Work out the finished part from the listing and answer in its coordinate system (mm). Face numbers are marked on the shaded views. A direction names the side the tool comes from. Give positions to 0.01 mm unless a question says otherwise; leave off trailing zeros. Loops run counter-clockwise (first coordinate to the right, second up) from the corner with the lowest first, then second, coordinate; pieces in that order, holes last. Notation, with made-up numbers: (-20.5, 16) - (16.5, 16) arc R21 cw to (16.5, 21) - close; hole circle Ø5 at (15.5, 85.5). An arc over 180 degrees is marked (long way). One line per question, with ' | ' between items. Start each with the question number.
1. Find the intervals of material crossed by line 1 (Y direction, x = 3.75, z = 0.65); line 2 (Y direction, x = 7.75, z = 1.4); line 3 (Y direction, x = 7.25, z = 2.8), in increasing order.
2. For a pull along Y with two mould halves and no side action, classify the marked faces 4, 5 and 6 as released by +Y, released by -Y, zero draft, split by the parting line, or undercut.
3. Which of the six approach directions +Z, -Z, +X, -X, +Y, -Y give full straight-line access (tool end or side, diameter ignored) to the marked faces 1, 2 and 3?
4. Section C-C (y = 9) is taken. Determine the outline of the cut face in (x, z).
5. Section A-A (x = 4) is taken. Determine the outline of the cut face in (y, z).
6. Section D-D (x = 0.25) is taken. Determine the outline of the cut face in (y, z).
7. Each of these flat-tipped pins is pushed along its axis until it touches: pin 1 (2 mm diameter, centred on x = -3, y = -3.5, fed in from +Z); pin 2 (1.5 mm diameter, centred on x = -6.5, z = 2, fed in from +Y); pin 3 (1.6 mm diameter, centred on y = -3.5, z = 1.5, fed in from +X). Where does it stop, or does it pass through?
Autodesk Inventor part; units mm, degrees
ref_plane "YZ Plane" through (0, 0, 0) normal (1, 0, 0) x (0, 1, 0)
ref_plane "XZ Plane" through (0, 0, 0) normal (0, 1, 0) x (-1, 0, 0)
ref_plane "XY Plane" through (0, 0, 0) normal (0, 0, 1) x (1, 0, 0)
sketch "Sketch1" plane through (0, 0, 0) normal (0, 0, 1) x (1, 0, 0)
  line L0 (-8.4, 0) -> (8.4, 0) construction
  line L1 (0, -20.65) -> (0, 20.65) construction
  line L2 (6, -14.75) -> (-6, -14.75)
  line L3 (-6, -14.75) -> (-6, 14.75)
  line L4 (-6, 14.75) -> (6, 14.75)
  line L5 (6, 14.75) -> (6, -14.75)
  line L6 (6, -14.75) -> (-6, 14.75) construction
  line L7 (-6, -14.75) -> (6, 14.75) construction
  point P0 (0, 0)
  dimension "d0" = 12
  dimension "d1" = 29.5
extrude "Extrusion1" add sketch "Sketch1" along normal blind 2
sketch "Sketch3" plane through (-6, 14.75, 2) normal (0, 1, 0) x (1, 0, 0)
  line L0 (0, 2) -> (12, 2) construction
  line L1 (0, 2) -> (0, 0) construction
  line L2 (12, 0) -> (0, 0) construction
  circle A0 centre (0, 0.5) radius 1.5
  line L3 (12, 2) -> (12, 0)
  point P0 (6, 2)
  dimension "d7" = 3
extrude "Extrusion3" add sketch "Sketch3" against normal up to surface (29.5 mm away)
sketch "Sketch5" plane through (6, 14.75, 2) normal (0, 1, 0) x (1, 0, 0)
  arc A0 (-12, 2) -> (-10.5858, 0) centre (-12, 0.5) ccw construction
  line L0 (0, 0) -> (-10.5858, 0) construction
  line L1 (0, 2) -> (0, 0) construction
  line L2 (-12, 2) -> (0, 2) construction
  circle A1 centre (-12, 0.5) radius 1.5
  point P0 (-6, 2)
extrude "Extrusion5" add sketch "Sketch5" along normal blind 1
mirror "Mirror3" about plane through (0, 0, 0) normal (0, 1, 0) of "Extrusion5"
sketch "Sketch6" plane through (0, 0, 2) normal (0, 0, 1) x (1, 0, 0)
  line L0 (-4.5858, 14.75) -> (-4.5858, -14.75) construction
  line L1 (-4.5858, -14.75) -> (6, -14.75) construction
  line L2 (6, -14.75) -> (6, 14.75) construction
  line L3 (6, 14.75) -> (-4.5858, 14.75) construction
  line L4 (-9.1, 0) -> (12.6, 0) construction
  line L5 (-6, 14.75) -> (6, 14.75)
  line L6 (1, 14.75) -> (1, 16.75)
  line L7 (1, 16.75) -> (10.5, 16.75)
  line L8 (2.75, 15.5) -> (2.75, 14.75)
  line L9 (1, 14.75) -> (2.75, 14.75)
  line L10 (2.75, 15.5) -> (6.75, 15.5)
  line L11 (6.75, 15.5) -> (6.75, 14.75)
  line L12 (6.75, 14.75) -> (10.5, 14.75)
  line L13 (10.5, 16.75) -> (10.5, 14.75)
  line L14 (6, 14.75) -> (-4.5858, 14.75)
  line L15 (1, -14.75) -> (1, -16.75)
  line L16 (1, -16.75) -> (10.5, -16.75)
  line L17 (2.75, -15.5) -> (2.75, -14.75)
  line L18 (1, -14.75) -> (2.75, -14.75)
  line L19 (2.75, -15.5) -> (6.75, -15.5)
  line L20 (6.75, -15.5) -> (6.75, -14.75)
  line L21 (6.75, -14.75) -> (10.5, -14.75)
  line L22 (10.5, -16.75) -> (10.5, -14.75)
  line L23 (0, 14.75) -> (0, 17.3845) construction
  point P0 (0, 0)
  dimension "d14" = 2
  dimension "d15" = 0.75
  dimension "d16" = 0.75
  dimension "d17" = 1.75
  dimension "d18" = 4.5
  dimension "d40" = 1
extrude "Extrusion6" add sketch "Sketch6" against normal up to surface (2 mm away)
sketch "Skizze9" plane through (0, 0, 2) normal (0, 0, 1) x (1, 0, 0)
  line L0 (-4.5858, 14.75) -> (-4.5858, -14.75) construction
  line L1 (-4.5858, -14.75) -> (1, -14.75) construction
  line L2 (1, -14.75) -> (1, -16.75) construction
  line L3 (1, -16.75) -> (10.5, -16.75) construction
  line L4 (10.5, -16.75) -> (10.5, -14.75) construction
  line L5 (10.5, -14.75) -> (6.75, -14.75) construction
  line L6 (6.75, -14.75) -> (6.75, -15.5) construction
  line L7 (6.75, -15.5) -> (2.75, -15.5) construction
  line L8 (2.75, -15.5) -> (2.75, -14.75) construction
  line L9 (2.75, -14.75) -> (6, -14.75) construction
  line L10 (6, -14.75) -> (6, 14.75) construction
  line L11 (6, 14.75) -> (2.75, 14.75) construction
  line L12 (2.75, 14.75) -> (2.75, 15.5) construction
  line L13 (2.75, 15.5) -> (6.75, 15.5) construction
  line L14 (6.75, 15.5) -> (6.75, 14.75) construction
  line L15 (6.75, 14.75) -> (10.5, 14.75) construction
  line L16 (10.5, 14.75) -> (10.5, 16.75) construction
  line L17 (10.5, 16.75) -> (1, 16.75) construction
  line L18 (1, 16.75) -> (1, 14.75) construction
  line L19 (1, 14.75) -> (-4.5858, 14.75) construction
  line L20 (1, 14.75) -> (-4.5858, 14.75)
  line L21 (1, 16.75) -> (1, 14.75)
  line L22 (1, 14.75) -> (1, 16.75)
  line L23 (1, 16.75) -> (10.5, 16.75)
  line L24 (10.5, 14.75) -> (10.5, 16.75)
  line L25 (10.5, 16.75) -> (10.5, 14.75)
  line L26 (10.5, 14.75) -> (6.75, 14.75)
  line L27 (6.75, 15.5) -> (6.75, 14.75)
  line L28 (6.75, 14.75) -> (6.75, 15.5)
  line L29 (6.75, 15.5) -> (2.75, 15.5)
  line L30 (6.75, 15.5) -> (2.75, 15.5)
  line L31 (2.75, 14.75) -> (2.75, 15.5)
  line L32 (2.75, 15.5) -> (2.75, 14.75)
  line L33 (2.75, 14.75) -> (1, 14.75)
  line L34 (1, -16.75) -> (1, -14.75)
  line L35 (1, -14.75) -> (1, -16.75)
  line L36 (1, -16.75) -> (10.5, -16.75)
  line L37 (10.5, -16.75) -> (10.5, -14.75)
  line L38 (10.5, -16.75) -> (10.5, -14.75)
  line L39 (10.5, -14.75) -> (6.75, -14.75)
  line L40 (6.75, -14.75) -> (6.75, -15.5)
  line L41 (6.75, -14.75) -> (6.75, -15.5)
  line L42 (6.75, -15.5) -> (2.75, -15.5)
  line L43 (2.75, -15.5) -> (2.75, -14.75)
  line L44 (2.75, -14.75) -> (1, -14.75)
  point P0 (0, 0)
extrude "Extrusion9" add sketch "Skizze9" along normal blind 1
sketch "Skizze10" plane through (0, 0, 0) normal (0, 1, 0) x (-1, 0, 0)
  line L0 (-10.5, 0) -> (-1, 0) construction
  line L1 (-10.5, 0) -> (-10.5, 3) construction
  line L2 (-1, 3) -> (-10.5, 3) construction
  line L3 (-1, 0) -> (-1, 3) construction
  line L4 (-10.5, 0) -> (-6.75, 0) construction
  line L5 (-10.5, 0) -> (-10.5, 3) construction
  line L6 (-6.75, 3) -> (-10.5, 3) construction
  line L7 (-6.75, 0) -> (-6.75, 3) construction
  line L8 (-6.75, 1.5) -> (-10.5, 1.5) construction
  line L9 (-10.5, 3) -> (-1, 3) construction
  line L10 (-10.5, 0) -> (-6.75, 0) construction
  line L11 (-8.625, 0) -> (-8.625, 3) construction
  line L12 (-6.75, 3) -> (-10.5, 3) construction
  circle A0 centre (-8.625, 1.5) radius 1.6
  point P0 (0, 0)
  dimension "d32" = 3.2
extrude "Extrusion10" cut sketch "Skizze10" along normal mid plane 32
chamfer "Fase1" distance 6 distance2 1 1 edges at (1, 15.75, 3) measured on face at (6.5227, 16.5, 3)
chamfer "Fase2" distance 6 distance2 1 1 edges at (1, -15.75, 3) measured on face at (6.5227, -16.5, 3)
fillet "Rundung1" radius 2 2 edges at (1, 16.75, 1) (1, -16.75, 1)
properties part number "20_Rect_Aperture_door_hinge"
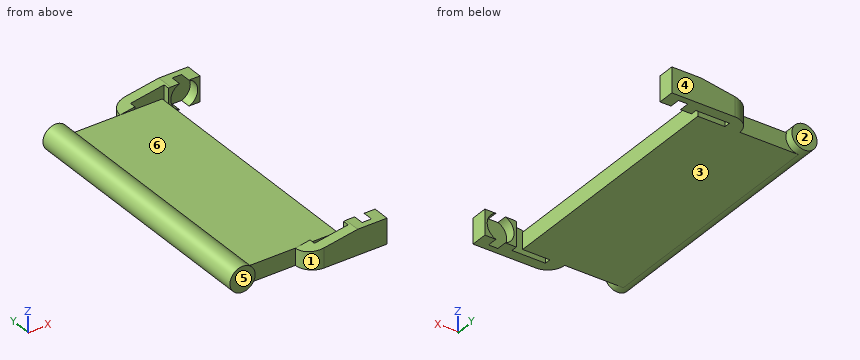
Conclusion:
1) line 1: -16.75 to -15.5, -14.75 to 14.75, 15.5 to 16.75 | line 2: -16.75 to -16, 16 to 16.75 | line 3: -16.75 to -14.75, 14.75 to 16.75
2) face 4: released by +Y | face 5: released by -Y | face 6: undercut
3) face 1: +Z, -Z, -Y | face 2: +Z, -Z, -X, +Y | face 3: -Z, +X, -X, +Y, -Y
4) outline: (-6, 0) - (6, 0) - (6, 2) - (-4.59, 2) arc R1.5 ccw (long way) to start
5) outline: (-16.75, 0) - (-15.5, 0) - (-15.5, 2.5) - (-16.75, 2.5) - close; (-14.75, 0) - (14.75, 0) - (14.75, 2) - (-14.75, 2) - close; (15.5, 0) - (16.75, 0) - (16.75, 2.5) - (15.5, 2.5) - close
6) outline: (-14.75, 0) - (14.75, 0) - (14.75, 2) - (-14.75, 2) - close
7) pin 1: z = 2 | pin 2: y = 15.75 | pin 3: x = 6
